CAD build for the part. Positions are in the model's coordinates, mm. Coordinates: 2 decimals unless noted, no trailing zeros. Order: outer loops, then holes, each group sorted by start corner. A loop starts at its lowest first (then second) coordinate and runs counter-clockwise, first axis right, second up. Notation, with made-up numbers: (-39, 88) - (8, 88) arc R21 cw to (8, 127) - close; hole circle Ø3 at (88, -34.5). An arc over 180 degrees is marked (long way). Write each question's results on one line, items separated by ' | '. Start each with the question number.
Q1. Wall check: probe 1 along X at (y, z) = (1.45, 19); probe 2 along Z at (x, y) = (56, 0.25) (3 decimals); probe 3 along X at (y, z) = (0.7, 37.5). Give the ranges that are in metal, low to high.
Q2. Band-saw the part on D-D, the plane y = 0.85. Count the separate pieces of the cut face and the enclosed holes in it, then the cut area to 3 significant figures.
Q3. Band-saw the part on B-B, the plane x = 57.15. Write the cut outline in (y, z) (3 decimals).
Q4. Pin check, flat tip, straight feed: P1, Ø4.5, axis at x = -2.27, z = 19.05, coming from the +Y side (3 decimals). Stop position of the tip, or through.
Q5. Band-saw the part on A-A, the plane z = 44.45. Write the cut outline in (x, y) (3 decimals), then the cut area to 3 significant figures.
Q6. Band-saw the part on C-C, the plane x = 14. Write the cut outline in (y, z) (3 decimals), then the cut area to 3 significant figures.
```python
from build123d import *

# Parameters (mm, degrees)
BASEWITH_ALIGNMENT_W = 76.2
BASEWITH_ALIGNMENT_H = 76.2
BASEWITH_ALIGNMENT_R = 3.175
BOSS_EXTRUDE1_DEPTH  = 3.175
CUT_EXTRUDE6_DEPTH   = 88.643803261
LPATTERN1_COUNT      = 8
LPATTERN1_PITCH      = 6.35
LPATTERN1_COUNT_DIR2 = 3
LPATTERN1_PITCH_DIR2 = 25.4


with BuildPart() as part:
    # BaseWith Alignment → Boss-Extrude1 (new body)
    with BuildSketch(Plane(origin=(0, 0, 0), x_dir=(1, 0, 0), z_dir=(0, 1, 0))):
        with Locations((25.4, -22.225)):
            Rectangle(BASEWITH_ALIGNMENT_W, BASEWITH_ALIGNMENT_H)
        with Locations(Location((-6.35, 9.525, 0), (0, 0, 270))):
            Circle(BASEWITH_ALIGNMENT_R, mode=Mode.SUBTRACT)
        with Locations(Location((57.15, 9.525, 0), (0, 0, 270))):
            Circle(BASEWITH_ALIGNMENT_R, mode=Mode.SUBTRACT)
        with Locations(Location((-6.35, -53.975, 0), (0, 0, 270))):
            Circle(BASEWITH_ALIGNMENT_R, mode=Mode.SUBTRACT)
        with Locations(Location((57.15, -53.975, 0), (0, 0, 270))):
            Circle(BASEWITH_ALIGNMENT_R, mode=Mode.SUBTRACT)
        with Locations(Location((12.7, -22.225, 0), (0, 0, 270))):
            Circle(BASEWITH_ALIGNMENT_R, mode=Mode.SUBTRACT)
        with Locations(Location((38.1, -22.225, 0), (0, 0, 270))):
            Circle(BASEWITH_ALIGNMENT_R, mode=Mode.SUBTRACT)
    extrude(amount=BOSS_EXTRUDE1_DEPTH)

    # Sketch1 → Cut-Extrude6 (cut, through all)
    with BuildSketch(Plane(origin=(0, 0, 0), x_dir=(-1, 0, 0), z_dir=(0, -1, 0))):
        with BuildLine():
            Line((2.017857143, -1.961432458), (-3.110714286, -1.296526148))
            ThreePointArc((-3.110714286, -1.296526148), (-4.25, 0), (-3.110714286, 1.296526148))
            Line((-3.110714286, 1.296526148), (2.017857143, 1.961432458))
            ThreePointArc((2.017857143, 1.961432458), (4.25, 0), (2.017857143, -1.961432458))
        make_face()
    cut_extrude6 = extrude(amount=-CUT_EXTRUDE6_DEPTH, mode=Mode.SUBTRACT)

    # LPattern1: Cut-Extrude6 8 × 3
    with Locations(*[(j * LPATTERN1_PITCH_DIR2, 0, i * LPATTERN1_PITCH) for i in range(LPATTERN1_COUNT) for j in range(LPATTERN1_COUNT_DIR2) if (i, j) != (0, 0)]):
        add(cut_extrude6, mode=Mode.SUBTRACT)


solid = part.part
```
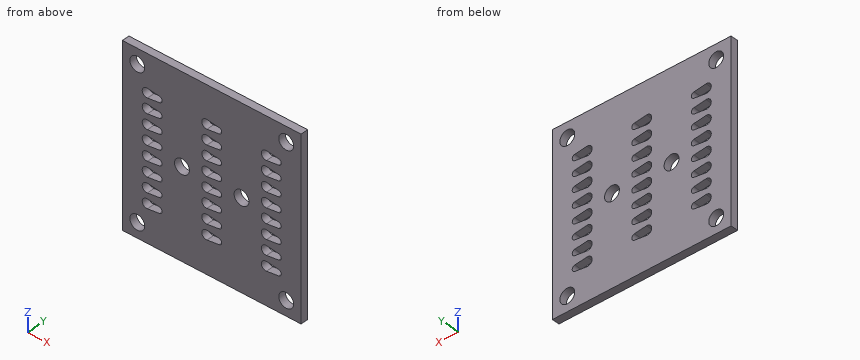
Results below:
1) probe 1: x = -12.7 to -4.25, 4.25 to 21.15, 29.65 to 46.55, 55.05 to 63.5 | probe 2: z = -15.875 to -12.484, -6.566 to 51.016, 56.934 to 60.325 | probe 3: x = -12.7 to -4.16, 4.1 to 21.24, 29.5 to 46.64, 54.9 to 63.5
2) separate pieces: 1 | enclosed holes: 30 | area: 4,990 mm²
3) outline: (0, -15.875) - (3.175, -15.875) - (3.175, -12.7) - (0, -12.7) - close; (0, -6.35) - (3.175, -6.35) - (3.175, 50.8) - (0, 50.8) - close; (0, 57.15) - (3.175, 57.15) - (3.175, 60.325) - (0, 60.325) - close
4) P1: stops at y = 3.175
5) outline: (-12.7, 0) - (-4.25, 0) - (-4.25, 3.175) - (-12.7, 3.175) - close; (4.25, 0) - (21.15, 0) - (21.15, 3.175) - (4.25, 3.175) - close; (29.65, 0) - (46.55, 0) - (46.55, 3.175) - (29.65, 3.175) - close; (55.05, 0) - (63.5, 0) - (63.5, 3.175) - (55.05, 3.175) - close | area: 161 mm²
6) outline: (0, -15.875) - (3.175, -15.875) - (3.175, 19.328) - (0, 19.328) - close; (0, 25.122) - (3.175, 25.122) - (3.175, 60.325) - (0, 60.325) - close | area: 224 mm²
